from build123d import *

# Parameters (mm, degrees)
F1_DEPTH = 127
F2_T     = -7.62


with BuildPart() as f1:
    # F0 (on Top) → F1 (new body)
    with BuildSketch(Plane.XY):
        Polygon((-39.284959, 78.533807), (-85.893974, 18.25081), (-67.823074, -55.775419), (1.319984, -87.80162), (69.469067, -53.71141), (85.306526, 20.824587), (36.906431, 79.679246), align=None)
    extrude(amount=F1_DEPTH)

    # F2
    f2_openings = [f1.faces().sort_by_distance(p)[0] for p in [
        (0, 0, 127),
    ]]
    offset(amount=F2_T, openings=f2_openings)


solid = f1.part
Source: CAD feature listing. Evaluate the final solid. Frame: model axes, mm. A direction names the side the tool comes from. Round coordinates to 2 decimals unless told otherwise and drop trailing zeros. Loops run counter-clockwise (first coordinate to the right, second up) from the corner with the lowest first, then second, coordinate; pieces in that order, holes last.
Q1. Ray query, line 1 (X direction, y = -3.5, z = 53.5); line 2 (X direction, y = -78.5, z = 119); line 3 (Z direction, x = -71.5, y = 14). Return the intervals inside material, ascending.
Q2. Section A-A, the plane z = 91. Return loops of the section in (x, y).
Q3. Section B-B, the plane x = -9.5. Return loops of the section in (y, z), plus the area to 4 significant figures.
Q4. First-contact query: P1, Ø6, axis at y = 56.5, z = 47, coming from the -X side; P2, Ø4, axis at y = 24.5, z = 29, coming from the +X side; P3, Ø2, axis at x = -26.5, y = 18.5, coming from the +Z side. Flat tips, straight axial feed; report the tip coordinate or a pass-through.
Q5. Section C-C, the plane y = -43. Return loops of the section in (x, z).
Q6. Access query for faces 1 (the face through (31.55, -64.16, 66.47)), 2 (the face through (-70, -16, 127)). Directions: +Z, -Z, +X, -X, +Y, -Y. A direction counts if a zero-diameter tool reaches every point of the face in a straight line with its end or side. Return the directions, or none.
Q7. Mould query, pull axis Y, two halves, no side actions, for faces 3 (the face through (-76.985, -18.244, 62.611)), 4 (the face through (-1, -3, 0)), 5 (the face through (69.834, -15.331, 66.474)), 6 (the face through (-62.263, 48.814, 62.611)). Classes: pulls with the +Y half, pulls with the -Y half, needs draft (parallel to the pull), parting line crosses it, or undercut.
Solutions:
1. line 1: x = -80.58 to -72.74, 72.35 to 80.14
1. line 2: x = -18.76 to -0.63, 2.88 to 19.91
1. line 3: z = 0 to 7.62
2. outline: (-85.89, 18.25) - (-67.82, -55.78) - (1.32, -87.8) - (69.47, -53.71) - (85.31, 20.82) - (36.91, 79.68) - (-39.28, 78.53) - close; hole (-77.62, 16.49) - (-61.29, -50.4) - (1.19, -79.35) - (62.78, -48.54) - (77.09, 18.82) - (33.35, 72) - (-35.5, 70.97) - close
3. outline: (-82.79, 0) - (78.98, 0) - (78.98, 127) - (71.36, 127) - (71.36, 7.62) - (-74.39, 7.62) - (-74.39, 127) - (-82.79, 127) - close
3. area: 3,145 mm2
4. P1: stops at x = -58.64
4. P2: stops at x = 83.93
4. P3: stops at z = 7.62
5. outline: (-70.94, 0) - (71.75, 0) - (71.75, 127) - (63.95, 127) - (63.95, 7.62) - (-63.1, 7.62) - (-63.1, 127) - (-70.94, 127) - close
6. face 1: +Z
6. face 2: +Z, +X, -X, +Y, -Y
7. face 3: pulls with the -Y half
7. face 4: needs draft
7. face 5: undercut
7. face 6: pulls with the +Y half
